from build123d import *

# Parameters (mm, degrees)
BOSS_EXTRUDE2_DEPTH  = 25.4
M5_CLEARANCE_HOLE2_D = 5.5


with BuildPart() as part:
    # Sketch1<3> → Boss-Extrude2 (new body)
    with BuildSketch(Plane.XY):
        with BuildLine():
            Line((13.452137377, 6.35), (50.8, 6.35))
            Line((50.8, 6.35), (50.8, 19.05))
            Line((50.8, 19.05), (24.85, 19.05))
            ThreePointArc((24.85, 19.05), (0, 43.9), (-24.85, 19.05))
            Line((-24.85, 19.05), (-50.8, 19.05))
            Line((-50.8, 19.05), (-50.8, 6.35))
            Line((-50.8, 6.35), (-13.452137377, 6.35))
            ThreePointArc((-13.452137377, 6.35), (0, 37.55), (13.452137377, 6.35))
        make_face()
    extrude(amount=BOSS_EXTRUDE2_DEPTH)

    # M5 Clearance Hole2 (through all)
    with Locations(Plane(origin=(0, 19.05, 0), x_dir=(1, 0, 0), z_dir=(0, 1, 0))):
        with Locations((38.1, -12.7), (-38.1, -12.7)):
            Hole(M5_CLEARANCE_HOLE2_D / 2)


solid = part.part
Model file for the job. Use its own axes, mm. A direction names the side the tool comes from. Round coordinates to 2 decimals unless told otherwise and drop trailing zeros. Loops run counter-clockwise (first coordinate to the right, second up) from the corner with the lowest first, then second, coordinate; pieces in that order, holes last. Notation, with made-up numbers: (2.5, 53.25) -> (12.5, 53.25) arc R20 cw to (12.5, 65.25) -> close; hole circle Ø6 at (24, 62). An arc over 180 degrees is marked (long way). Answer as CSV lines item,"result". Start each with the question number.
1) Slice it at A-A (x = 38.1). List the corners of the cut face in (y, z).
2) Slice it at D-D (z = 20.75). List the corners of the cut face in (x, y), plus the area to 3 significant figures.
3) Probe line 1 along X through (y, z) = (18.5, 24); line 2 along Z through (x, y) = (-38.1, 12.5); line 3 along X through (y, z) = (12.5, 12.7). List the from-to ranges inside material, lowest first.
4) Tool access for faces 4 (the face through (38.696, 12.611, 15.385)), 5 (the face through (-37.6, 19.05, 9.7)), 6 (the face through (38, 19.05, 9.7)): list every direction of +Z, -Z, +X, -X, +Y, -Y with a clear straight run to the whole face (end or side of a thin tool).
5) Mould opens along X. For faces 1 (the face through (0, 38, 0)), 2 (the face through (50.8, 13, 13)), 3 (the face through (-35.918, 12.611, 14.373)) say: +X half, -X half, draft (parallel to the pull), parting line (faces both ways), or undercut.
6) Slice it at B-B (z = 12.7). List the corners of the cut face in (x, y).
7) Pin check, flat tips, straight feed: P1, Ø3.5, axis at x = 38.1, z = 12.7, coming from the -Y side; P2, Ø8, axis at x = 20, z = 16, coming from the +Y side; P3, Ø6, axis at x = 18, z = 8.5, coming from the +Y side; P4, Ø3, axis at y = 33, z = 12, coming from the +X side. Stop position of each tip, or through.
8) Slice it at C-C (y = 10.5). List the corners of the cut face in (x, z), plus the area to 3 significant figures.
Filled in:
1,outline,"(6.35, 0) -> (19.05, 0) -> (19.05, 9.95) -> (6.35, 9.95) -> close; (6.35, 15.45) -> (19.05, 15.45) -> (19.05, 25.4) -> (6.35, 25.4) -> close"
2,outline,"(-50.8, 6.35) -> (-13.45, 6.35) arc R18.5 cw (long way) to (13.45, 6.35) -> (50.8, 6.35) -> (50.8, 19.05) -> (24.85, 19.05) arc R24.85 ccw to (-24.85, 19.05) -> (-50.8, 19.05) -> close"
2,area,"1,290 mm2"
3,line 1,"x = -50.8 to -18.49, 18.49 to 50.8"
3,line 2,"z = 0 to 9.95, 15.45 to 25.4"
3,line 3,"x = -50.8 to -40.85, -35.35 to -17.3, 17.3 to 35.35, 40.85 to 50.8"
4,face 4,"+Y, -Y"
4,face 5,"+Z, -Z, -X, +Y"
4,face 6,"+Z, -Z, +X, +Y"
5,face 1,"draft"
5,face 2,"+X half"
5,face 3,"undercut"
6,outline,"(-50.8, 6.35) -> (-40.85, 6.35) -> (-40.85, 19.05) -> (-50.8, 19.05) -> close; (-35.35, 6.35) -> (-13.45, 6.35) arc R18.5 cw (long way) to (13.45, 6.35) -> (35.35, 6.35) -> (35.35, 19.05) -> (24.85, 19.05) arc R24.85 ccw to (-24.85, 19.05) -> (-35.35, 19.05) -> close; (40.85, 6.35) -> (50.8, 6.35) -> (50.8, 19.05) -> (40.85, 19.05) -> close"
7,P1,"passes through"
7,P2,"stops at y = 38.06"
7,P3,"stops at y = 38.86"
7,P4,"stops at x = 21.51"
8,outline,"(-50.8, 0) -> (-16.41, 0) -> (-16.41, 25.4) -> (-50.8, 25.4) -> close; (16.41, 0) -> (50.8, 0) -> (50.8, 25.4) -> (16.41, 25.4) -> close; hole circle Ø5.5 at (-38.1, 12.7); hole circle Ø5.5 at (38.1, 12.7)"
8,area,"1,700 mm2"
